from build123d import *

# Parameters (mm, degrees)
F1_DEPTH = 9.144
F2_W     = 2.06375
F2_H     = 2.0955
F2_W_2   = 2.2225
F2_H_2   = 1.11125
F2_H_3   = 2.413
F3_DEPTH = 5.08
F4_DEPTH = 15.24
F5_R     = 2.54


with BuildPart() as f1:
    # F0 (on Top) → F1 (new body)
    with BuildSketch(Plane.XY):
        Polygon((23.622, 2.749807667), (10.287, 4.5246649534), (10.287, -4.5246649534), (23.622, -2.749807667), align=None)
        Polygon((6.3920377387, 12.065), (0, 14.605), (0, -14.605), (6.3920377387, -12.065), (10.287, -4.5246649534), (10.287, 4.5246649534), align=None)
    extrude(amount=F1_DEPTH)

    # F2 (on face) → F3 (cut)
    with BuildSketch(Plane(origin=(0, 0, 0), x_dir=(0, -1, 0), z_dir=(-1, 0, 0))):
        with Locations((-2.143125, 4.572)):
            Rectangle(F2_W, F2_H)
        with Locations((0, 4.572)):
            Rectangle(F2_W_2, F2_H)
        with Locations((0, 2.968625)):
            Rectangle(F2_W_2, F2_H_2)
        with Locations((2.143125, 4.572)):
            Rectangle(F2_W, F2_H)
        with Locations((0, 6.175375)):
            Rectangle(F2_W_2, F2_H_2)
        with Locations((0, 1.2065)):
            Rectangle(F2_W_2, F2_H_3)
        with Locations((0, 7.9375)):
            Rectangle(F2_W_2, F2_H_3)
    extrude(amount=-F3_DEPTH, mode=Mode.SUBTRACT)

    # F2 (on face) → F4 (cut)
    with BuildSketch(Plane(origin=(0, 0, 0), x_dir=(0, -1, 0), z_dir=(-1, 0, 0))):
        with Locations((0, 2.968625)):
            Rectangle(F2_W_2, F2_H_2)
        with Locations((0, 4.572)):
            Rectangle(F2_W_2, F2_H)
        with Locations((0, 6.175375)):
            Rectangle(F2_W_2, F2_H_2)
    extrude(amount=-F4_DEPTH, mode=Mode.SUBTRACT)

    # F5
    f5_edges = [f1.edges().sort_by_distance(p)[0] for p in [
        (23.622, 2.749808, 4.572),
        (23.622, -2.749808, 4.572),
        (10.287, 4.524665, 4.572),
        (6.392038, 12.065, 4.572),
        (10.287, -4.524665, 4.572),
        (6.392038, -12.065, 4.572),
    ]]
    fillet(f5_edges, radius=F5_R)


solid = f1.part
Can you work these out from the model? Positions are in its coordinate system, mm. A direction names the side the tool comes from. Round coordinates to 2 decimals unless told otherwise and drop trailing zeros. Write each loop counter-clockwise with the first axis right and the second up, starting at its lowest first coordinate (ties: lowest second). Pieces come first, ordered by that corner, then holes. Notation, with made-up numbers: M -25.75,22 L -8.75,22 A21 cw -8.75,29 Z; hole C -14.75,48.5 d4. An arc over 180 degrees is marked long. Use a Markdown table: item, result.
Item 1: Which directions (+Z, -Z, +X, -X, +Y, -Y) give clear straight access to the entire face, cutting with the end or side of a thin tool? Please do faces 1 (the face through (5.08, 2, 5)), 2 (the face through (5.08, 0, 1)), 3 (the face through (6.267, -11.946, 4.636)).
Found:
| item | result |
|---|---|
| face 1 | -X |
| face 2 | +Z, -Z, -X |
| face 3 | +Z, -Z, +X, -Y |
Item 2: I want a section at C-C (x = 2.5). List the corners of the cut face in (y, z) for me (3 decimals).
Found:
| item | result |
|---|---|
| outline | M -13.612,0 L -1.111,0 L -1.111,3.524 L -3.175,3.524 L -3.175,5.62 L -1.111,5.62 L -1.111,9.144 L -13.612,9.144 Z; M 1.111,0 L 13.612,0 L 13.612,9.144 L 1.111,9.144 L 1.111,5.62 L 3.175,5.62 L 3.175,3.524 L 1.111,3.524 Z |
Item 3: For pin 1 Ø0.7 at (y, z) = (-0.5, 2) entering from -X; pin 2 Ø4.5 at (x, z) = (4, 3) entering from -Y; pin 3 Ø2.5 at (y, z) = (0.5, 5) entering from -X; pin 4 Ø3 at (x, z) = (10.5, 4.5) entering from +Y, each with a flat end and sliding along its axis, tell me the tip position at first contact or that it passes through.
Found:
| item | result |
|---|---|
| pin 1 | stops at x = 5.08 |
| pin 2 | stops at y = -13.91 |
| pin 3 | stops at x = 0 |
| pin 4 | stops at y = 7.02 |
Item 4: I want a section at B-B (x = 11.25). List the corners of the cut face in (y, z) for me, and give its area (3 significant figures).
Found:
| item | result |
|---|---|
| outline | M -4.42,0 L 4.42,0 L 4.42,9.14 L -4.42,9.14 Z; hole M -1.11,2.41 L 1.11,2.41 L 1.11,6.73 L -1.11,6.73 Z |
| area | 71.3 mm2 |
Item 5: I want a section at D-D (y = 6.75). List the corners of the cut face in (x, z) for me, and give its area (3 significant figures).
Found:
| item | result |
|---|---|
| outline | M 0,0 L 9.14,0 L 9.14,9.14 L 0,9.14 Z |
| area | 83.6 mm2 |
Item 6: We'd pull the mould along Y, two halves only. Please class faces 4 (the face through (9, 0, 9.144)), 5 (the face through (10.49, 4.78, 4.64)), 6 (the face through (3, 2, 5.62)): released by +Y, released by -Y, zero draft, split by the parting line, or undercut.
Found:
| item | result |
|---|---|
| face 4 | zero draft |
| face 5 | released by +Y |
| face 6 | undercut |
Item 7: If I drill on line 1 along Z through (x, y) = (13.75, 0.25); line 2 along X through (y, z) = (0.5, 0.5); line 3 along Y through (x, z) = (3, 2.5), over which ranges is the centre line in solid material (lowest first)? Write a range as [from, to].
Found:
| item | result |
|---|---|
| line 1 | z = [0, 2.41], [6.73, 9.14] |
| line 2 | x = [5.08, 23.62] |
| line 3 | y = [-13.41, -1.11], [1.11, 13.41] |
Item 8: I want a section at A-A (z = 8). List the corners of the cut face in (x, y) for me (3 decimals), and give its area (3 significant figures).
Found:
| item | result |
|---|---|
| outline | M 0,-14.605 L 5.509,-12.416 A2.54 ccw 6.828,-11.221 L 9.679,-5.702 A2.54 cw 11.6,-4.35 L 21.417,-3.043 A2.54 ccw 23.622,-0.525 L 23.622,0.525 A2.54 ccw 21.417,3.043 L 11.6,4.35 A2.54 cw 9.679,5.702 L 6.828,11.221 A2.54 ccw 5.509,12.416 L 0,14.605 L 0,1.111 L 5.08,1.111 L 5.08,-1.111 L 0,-1.111 Z |
| area | 319 mm2 |
